Can you work these out from the model? Positions are in its coordinate system, mm. A direction names the side the tool comes from. Round coordinates to 2 decimals unless told otherwise and drop trailing zeros. Write each loop counter-clockwise with the first axis right and the second up, starting at its lowest first coordinate (ties: lowest second). Pieces come first, ordered by that corner, then holes. Notation, with made-up numbers: (64.5, 5) - (97.5, 5) arc R28 cw to (97.5, 36) - close; hole circle Ø1 at (67, -8). An arc over 180 degrees is marked (long way). One line per item, written item: value. Start each with the question number.
(1) If I drill on L1, parallel to Y at x = 42, z = 2; L2, parallel to Y at x = 12, z = 1.7; L3, parallel to X at y = -25.5, z = 28.5, over which ranges is the centre line in solid material (lowest first)? Write a range as from..to.
(2) I want a section at A-A on y = -39.5. List the corners of the cut face in (x, z) for me, plus the area to 3 significant figures.
(3) I'm going to push flat-ended pins straight in: pin 1 Ø1.5 at (x, y) = (10, -32) entering from +Z; pin 2 Ø1.2 at (x, z) = (53, 29) entering from +Y; pin 3 Ø10 at (x, z) = (37, 47.5) entering from +Y; pin 4 Ø1.2 at (x, y) = (24.5, -1) entering from +Z. Where does each tip first touch, or does it pass through?
(4) I want a section at C-C on z = 47. List the corners of the cut face in (x, y) for me, plus the area to 3 significant figures.
(5) On a 3-axis mill with a long thin cutter (end or side, diameter ignored), from which of +Z, -Z, +X, -X, +Y, -Y can I reach the whole of each face in a straight line? I mean faces 1 (the face through (53, -24, 30)), 2 (the face through (27, -1, 11)), 3 (the face through (1.5, -24, 28)), 4 (the face through (27, -49, 26)). Say none if no direction works.
(6) I want a section at D-D on y = -28. List the corners of the cut face in (x, z) for me, plus the area to 3 significant figures.
(7) Thinking about a two-plate mould opening in X: for faces 5 (the face through (29.1, 0, 10.7)), 6 (the face through (54, -25, 26)), 7 (the face through (27, -47.5, 28)), which applies, +X half, -X half, draft (parallel to the pull), parting line (faces both ways), or undercut?
(8) I want a section at B-B on x = 12. List the corners of the cut face in (y, z) for me.
from build123d import *

# Parameters (mm, degrees)
SKETCH_W     = 54
SKETCH_H     = 49
SKETCH_R     = 3.5
SKETCH_R_2   = 4
PAD_DEPTH    = 3
PAD001_DEPTH = 50
SKETCH002_W  = 5
SKETCH002_H  = 45
POCKET_DEPTH = 1.5
SKETCH003_W  = 51
SKETCH003_H  = 1.5
PAD002_DEPTH = 8


with BuildPart() as part:
    # Sketch → Pad (new body)
    with BuildSketch(Plane.XY):
        with Locations((27, -24.5)):
            Rectangle(SKETCH_W, SKETCH_H)
        with Locations((12, -39.5)):
            Circle(SKETCH_R, mode=Mode.SUBTRACT)
        with Locations((42, -9.5)):
            Circle(SKETCH_R, mode=Mode.SUBTRACT)
        with Locations((12, -9.5)):
            Circle(SKETCH_R_2, mode=Mode.SUBTRACT)
        with Locations((42, -39.5)):
            Circle(SKETCH_R_2, mode=Mode.SUBTRACT)
    extrude(amount=PAD_DEPTH)

    # Sketch001 → Pad001 (new body)
    with BuildSketch(Plane.XY.offset(3)):
        Polygon((0, 0), (0, -49), (54, -49), (54, 0), (52.5, 0), (52.5, -47.5), (1.5, -47.5), (1.5, 0), align=None)
    extrude(amount=PAD001_DEPTH)

    # Sketch002 → Pocket (cut)
    with BuildSketch(Plane.YZ.offset(54)):
        with Locations((-21.5, 30.5)):
            Rectangle(SKETCH002_W, SKETCH002_H)
    extrude(amount=-POCKET_DEPTH, mode=Mode.SUBTRACT)

    # Sketch003 → Pad002 (new body)
    with BuildSketch(Plane.XY.offset(3)):
        with Locations((27, -0.75)):
            Rectangle(SKETCH003_W, SKETCH003_H)
    extrude(amount=PAD002_DEPTH)


solid = part.part
Established:
1. L1: -49..-43.5, -35.5..-13, -6..0
1. L2: -49..-43, -36..-13.5, -5.5..0
1. L3: 0..1.5, 52.5..54
2. outline: (0, 0) - (8.5, 0) - (8.5, 3) - (1.5, 3) - (1.5, 53) - (0, 53) - close; (15.5, 0) - (38, 0) - (38, 3) - (15.5, 3) - close; (46, 0) - (54, 0) - (54, 53) - (52.5, 53) - (52.5, 3) - (46, 3) - close
2. area: 267 mm2
3. pin 1: z = 3
3. pin 2: y = 0
3. pin 3: y = -47.5
3. pin 4: z = 11
4. outline: (0, -49) - (54, -49) - (54, -24) - (52.5, -24) - (52.5, -47.5) - (1.5, -47.5) - (1.5, 0) - (0, 0) - close; (52.5, -19) - (54, -19) - (54, 0) - (52.5, 0) - close
4. area: 216 mm2
5. face 1: +Z, +X
5. face 2: +Z, +Y
5. face 3: +Z
5. face 4: +Z, -Z, +X, -X, -Y
6. outline: (0, 0) - (54, 0) - (54, 53) - (52.5, 53) - (52.5, 3) - (1.5, 3) - (1.5, 53) - (0, 53) - close
6. area: 312 mm2
7. face 5: draft
7. face 6: +X half
7. face 7: undercut
8. outline: (-49, 0) - (-43, 0) - (-43, 3) - (-47.5, 3) - (-47.5, 53) - (-49, 53) - close; (-36, 0) - (-13.5, 0) - (-13.5, 3) - (-36, 3) - close; (-5.5, 0) - (0, 0) - (0, 11) - (-1.5, 11) - (-1.5, 3) - (-5.5, 3) - close
